from build123d import *

# Parameters (mm, degrees)
F0_R     = 8
F1_DEPTH = 24
F2_R     = 3
F3_DEPTH = 24.001
F5_D     = 2.5
F5_DEPTH = 8.001
F7_D     = 2.5
F7_DEPTH = 8.0010001


with BuildPart() as f1:
    # F0 (on Front) → F1 (new body)
    with BuildSketch(Plane.XZ):
        Circle(F0_R)
    extrude(amount=F1_DEPTH)

    # F2 (on Front) → F3 (cut, through all)
    with BuildSketch(Plane.XZ):
        Circle(F2_R)
    extrude(amount=F3_DEPTH, mode=Mode.SUBTRACT)

    # F5 (through all, one way)
    with BuildSketch(Plane.YZ):
        with Locations((-18, 0), (-6, 0)):
            Circle(F5_D / 2)
    extrude(amount=-F5_DEPTH, mode=Mode.SUBTRACT)

    # F7 (through all, one way)
    with BuildSketch(Plane.XY):
        with Locations((0, -18), (0, -6)):
            Circle(F7_D / 2)
    extrude(amount=-F7_DEPTH, mode=Mode.SUBTRACT)


solid = f1.part
Source: CAD feature listing. Evaluate the final solid. Frame: model axes, mm. A direction names the side the tool comes from. Give positions to 0.01 mm unless a question says otherwise; leave off trailing zeros. Write each loop counter-clockwise with the first axis right and the second up, starting at its lowest first coordinate (ties: lowest second). Pieces come first, ordered by that corner, then holes. Notation, with made-up numbers: (14.5, -8.5) - (68.5, -8.5) arc R21 cw to (68.5, 7.5) - close; hole circle Ø3 at (45.25, 42). An arc over 180 degrees is marked (long way). Write item = value, one per line. Start each with the question number.
Q1. Cut plane B-B, the plane x = 0. Return loops of the section in (y, z), then the cut area to 3 significant figures.
Q2. Cut plane C-C, the plane y = -6. Return loops of the section in (x, z), then the cut area to 3 significant figures.
Q3. Pin query (flat end, axial travel): pin 1 Ø1.5 at (y, z) = (-3, 6) entering from -X; pin 2 Ø2 at (x, y) = (0, -6) entering from -Z; pin 3 Ø1 at (y, z) = (-4, 3.5) entering from +X. Return the tip coordinate at first contact, or that it passes through.
Q4. Cut plane D-D, the plane x = 2. Return loops of the section in (y, z), then the cut area to 3 significant figures.
Q5. Draft query along X for faces 1 (the cylindrical face through (1.19, -17.62, -5.33)), 2 (the cylindrical face through (1.155, -6.479, -5.328)), 3 (the cylindrical face through (7.39, -11.83, -3.06)), 4 (the cylindrical face through (-5.327, -16.845, -0.479)). Return one class per face: +X half, -X half, draft (parallel to the pull), parting line (faces both ways), or undercut.
Q6. Cut plane A-A, the plane z = 0. Return loops of the section in (x, y), then the cut area to 3 significant figures.
Q7. Reachability of faces 5 (the flat face through (3.4, -24, 0.1)), 6 (the cylindrical face through (-5.33, -4.81, 0.38)) from +Z, -Z, +X, -X, +Y, -Y: full face, straight path, thin tool, end or side. Return the list, or none.
Q8. Material intervals for probe 1 along Y at (x, z) = (0, -4.3); probe 2 along Z at (x, y) = (0, -9.5); probe 3 along Y at (x, z) = (0.5, -3.5), sorted ascending.
Computed values:
q1.outline = (-24, -8) - (-19.25, -8) - (-19.25, -3) - (-24, -3) - close; (-24, 3) - (0, 3) - (0, 8) - (-24, 8) - close; (-16.75, -8) - (-7.25, -8) - (-7.25, -3) - (-16.75, -3) - close; (-4.75, -8) - (0, -8) - (0, -3) - (-4.75, -3) - close
q1.area = 215 mm²
q2.outline = (-7.9, -1.25) arc R8 ccw to (-1.25, -7.9) - (-1.25, -2.73) arc R3 cw to (-2.73, -1.25) - close; (-7.9, 1.25) - (-2.73, 1.25) arc R3 cw (long way) to (1.25, -2.73) - (1.25, -7.9) arc R8 ccw (long way) to start
q2.area = 148 mm²
q3.pin_1 = -6.04
q3.pin_2 = 2.83
q3.pin_3 = 7.42
q4.outline = (-24, -7.75) - (0, -7.75) - (0, -2.24) - (-24, -2.24) - close; (-24, 2.24) - (0, 2.24) - (0, 7.75) - (-24, 7.75) - close
q4.area = 264 mm²
q5.face_1 = undercut
q5.face_2 = undercut
q5.face_3 = parting line
q5.face_4 = draft
q6.outline = (-8, -24) - (-3, -24) - (-3, -19.25) - (-8, -19.25) - close; (-8, -16.75) - (-3, -16.75) - (-3, -7.25) - (-8, -7.25) - close; (-8, -4.75) - (-3, -4.75) - (-3, 0) - (-8, 0) - close; (3, -24) - (8, -24) - (8, 0) - (3, 0) - close
q6.area = 215 mm²
q7.face_5 = +Z, -Z, +X, -X, -Y
q7.face_6 = -X
q8.probe_1 = -24 to -19.25, -16.75 to -7.25, -4.75 to 0
q8.probe_2 = -8 to -3, 3 to 8
q8.probe_3 = -24 to -19.15, -16.85 to -7.15, -4.85 to 0
